Part print with two shaded views. Sizes in mm from the minimum x, y, z corner. Round coordinates to 2 decimals unless told otherwise and drop trailing zeros. Order: outer loops, then holes, each group sorted by start corner. A loop starts at its lowest first (then second) coordinate and runs counter-clockwise, first axis right, second up. Notation, with made-up numbers: M 87,-35 L 123,-35 A37 ccw 123,4 Z; hole C -3,37 d7. An arc over 180 degrees is marked long. Put each result on its own line as item: value.
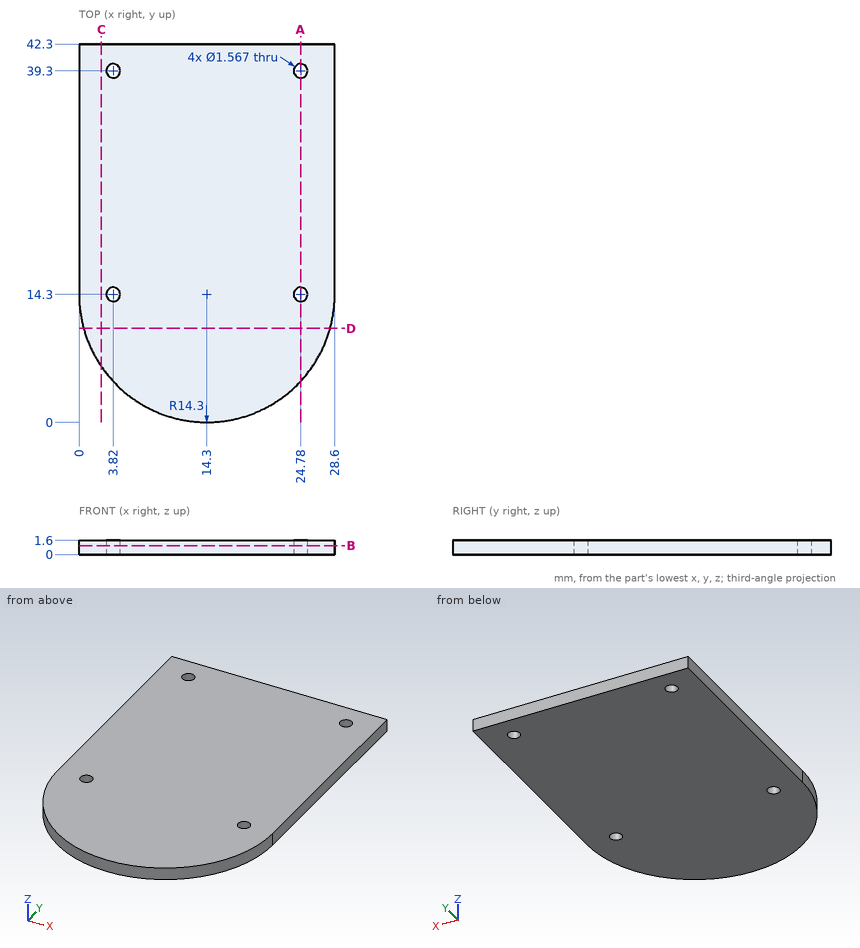
Item 1: Band-saw the part on A-A on x = 24.78. Give the cut face in (y, z), and give its area (3 significant figures).
Answers below:
outline: M 4.57,0 L 13.52,0 L 13.52,1.6 L 4.57,1.6 Z; M 15.08,0 L 38.52,0 L 38.52,1.6 L 15.08,1.6 Z; M 40.08,0 L 42.3,0 L 42.3,1.6 L 40.08,1.6 Z
area: 55.4 mm²
Item 2: Band-saw the part on C-C on x = 2.5. Give the cut face in (y, z).
Answers below:
outline: M 6.22,0 L 42.3,0 L 42.3,1.6 L 6.22,1.6 Z
Item 3: Band-saw the part on D-D on y = 10.5. Give the cut face in (x, z), and give its area (3 significant figures).
Answers below:
outline: M 0.51,0 L 28.09,0 L 28.09,1.6 L 0.51,1.6 Z
area: 44.1 mm²
Item 4: Pin check, flat tips, straight feed: P1, Ø10, axis at x = 11, y = 33, coming from the -Z side; P2, Ø1.3, axis at x = 3.82, y = 39.3, coming from the -Z side. Stop position of each tip, or through.
Answers below:
P1: z = 0
P2: through
Item 5: Probe line 1 along Y through (x, z) = (3.82, 1); line 2 along X through (y, z) = (40, 0.35); line 3 along Y through (x, z) = (14.25, 0.9). List the from-to ranges inside material, lowest first. Write a range as [from, to].
Answers below:
line 1: [4.57, 13.52], [15.08, 38.52], [40.08, 42.3]
line 2: [0, 3.47], [4.17, 24.43], [25.13, 28.6]
line 3: [0, 42.3]
Item 6: Band-saw the part on B-B on z = 1. Give the cut face in (x, y), and give its area (3 significant figures).
Answers below:
outline: M 0,14.3 A14.3 ccw 28.6,14.3 L 28.6,42.3 L 0,42.3 Z; hole C 3.82,14.3 d1.57; hole C 3.82,39.3 d1.57; hole C 24.78,14.3 d1.57; hole C 24.78,39.3 d1.57
area: 1,110 mm²
